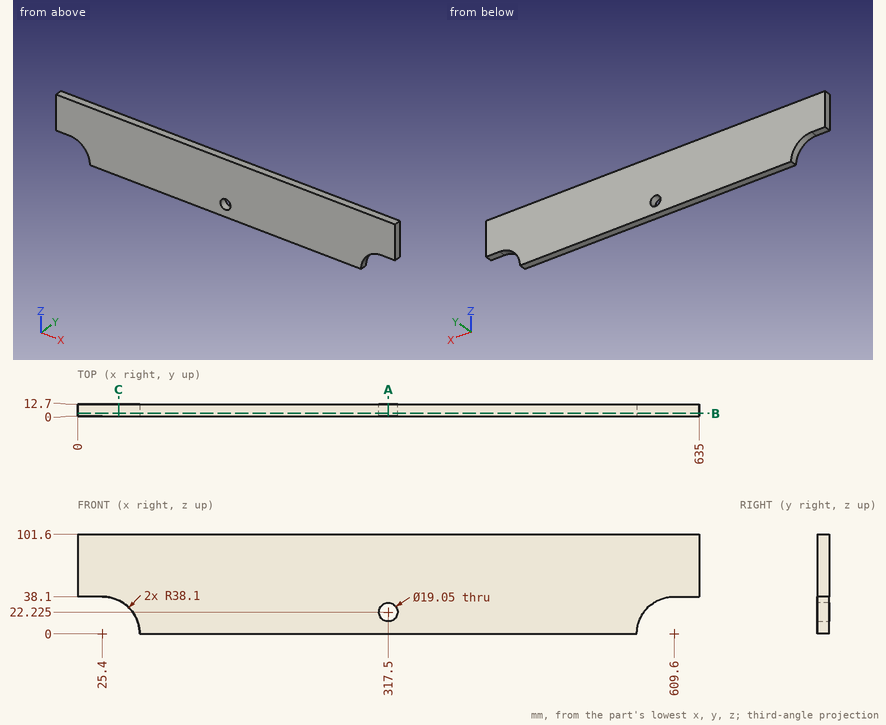
Geometry: see drawing. Coordinates: mm, zero at the bounding-box minimum. Coordinates: 2 decimals unless noted, no trailing zeros. Loops run counter-clockwise (first coordinate to the right, second up) from the corner with the lowest first, then second, coordinate; pieces in that order, holes last.
Q1. Cut plane B-B (y = 3). Output: boundary loops of the cut face in (x, z) (3 decimals).
Q2. Contact query for flat-ended pins moving along their axis: pin 1 (6.5 mm diameter, centred on x = 621, y = 8.5, fed in from -Z); pin 2 (11.5 mm diameter, centred on x = 317.5, z = 22.225, fed in from +Y); pin 3 (1 mm diameter, centred on y = 7, z = 17, fed in from -X). Output: stop coordinate, or through.
Q3. Cut plane C-C (x = 42). Output: boundary loops of the cut face in (y, z), then the cut area to 3 significant figures.
Q4. Cut plane A-A (x = 317.5). Output: boundary loops of the cut face in (y, z), then the cut area to 3 significant figures.
Q5. Material intervals for line 1 (X direction, y = 8.5, z = 21); line 2 (X direction, y = 6.25, z = 30.5); line 3 (X direction, y = 10.75, z = 34), sorted ascending.
Working result:
1. outline: (0, 38.1) - (25.4, 38.1) arc R38.1 cw to (63.5, 0) - (571.5, 0) arc R38.1 cw to (609.6, 38.1) - (635, 38.1) - (635, 101.6) - (0, 101.6) - close; hole circle Ø19.05 at (317.5, 22.225)
2. pin 1: stops at z = 38.1
2. pin 2: passes through
2. pin 3: stops at x = 59.24
3. outline: (0, 34.29) - (12.7, 34.29) - (12.7, 101.6) - (0, 101.6) - close
3. area: 855 mm2
4. outline: (0, 0) - (12.7, 0) - (12.7, 12.7) - (0, 12.7) - close; (0, 31.75) - (12.7, 31.75) - (12.7, 101.6) - (0, 101.6) - close
4. area: 1,050 mm2
5. line 1: x = 57.19 to 308.05, 326.95 to 577.81
5. line 2: x = 48.23 to 312.78, 322.22 to 586.77
5. line 3: x = 42.59 to 592.41
